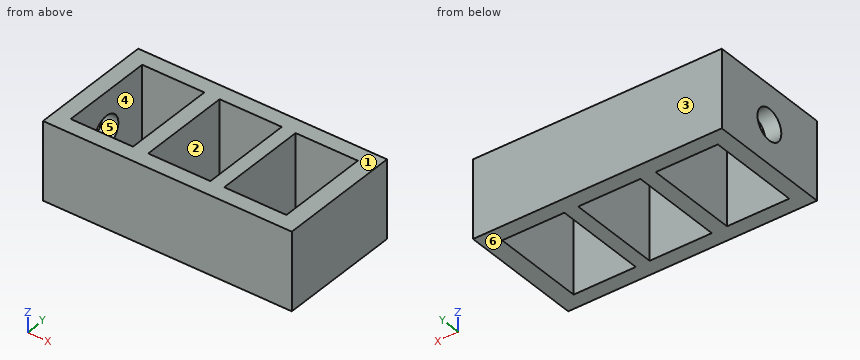
```python
from build123d import *

# Parameters (mm, degrees)
SKETCH_W     = 160
SKETCH_H     = 80
SKETCH_W_2   = 40
SKETCH_H_2   = 60
PAD_DEPTH    = 50
SKETCH001_R  = 10
POCKET_DEPTH = 11


with BuildPart() as part:
    # Sketch → Pad (new body)
    with BuildSketch(Plane.XY):
        Rectangle(SKETCH_W, SKETCH_H)
        with Locations((-49.803748, 0)):
            Rectangle(SKETCH_W_2, SKETCH_H_2, mode=Mode.SUBTRACT)
        Rectangle(SKETCH_W_2, SKETCH_H_2, mode=Mode.SUBTRACT)
        with Locations((48.892394, 0)):
            Rectangle(SKETCH_W_2, SKETCH_H_2, mode=Mode.SUBTRACT)
    extrude(amount=PAD_DEPTH)

    # Sketch001 (on Face1 of Pad) → Pocket (cut)
    with BuildSketch(Plane(origin=(-80, 0, 0), x_dir=(0, -1, 0), z_dir=(-1, 0, 0))):
        with Locations((0, 25)):
            Circle(SKETCH001_R)
    extrude(amount=-POCKET_DEPTH, mode=Mode.SUBTRACT)


solid = part.part
```
For this review, take the finished solid that the model builds, in its own axes (mm). Face numbers are marked on the shaded views. A direction names the side the tool comes from. Round coordinates to 2 decimals unless told otherwise and drop trailing zeros. Order: outer loops, then holes, each group sorted by start corner. A loop starts at its lowest first (then second) coordinate and runs counter-clockwise, first axis right, second up. Notation, with made-up numbers: (68, 76) -> (97, 76) arc R20 ccw to (97, 99) -> close; hole circle Ø9 at (16, -35.75). An arc over 180 degrees is marked (long way). Use a Markdown table: item, result.
Item 1: Draft analysis for pull direction Y (two halves, no side actions). For the marked faces 1, 2 and 3, state which applies: +Y half, -Y half, draft (parallel to the pull), parting line (faces both ways), or undercut.
Resolved:
| item | result |
|---|---|
| face 1 | draft |
| face 2 | undercut |
| face 3 | +Y half |
Item 2: For line 1 along X through (y, z) = (8.5, 43.5); line 2 along X through (y, z) = (0, 25.5); line 3 along Y through (x, z) = (31, 17), list the stretches that pass through material, from the lowest coordinate up. Write a range as [from, to].
Resolved:
| item | result |
|---|---|
| line 1 | x = [-80, -69.8], [-29.8, -20], [20, 28.89], [68.89, 80] |
| line 2 | x = [-29.8, -20], [20, 28.89], [68.89, 80] |
| line 3 | y = [-40, -30], [30, 40] |
Item 3: Take a section at D-D (x = -63.5). State the section outline as (y, z) points.
Resolved:
| item | result |
|---|---|
| outline | (-40, 0) -> (-30, 0) -> (-30, 50) -> (-40, 50) -> close; (30, 0) -> (40, 0) -> (40, 50) -> (30, 50) -> close |
Item 4: Take a section at A-A (z = 12). State the section outline as (x, y) points, plus the area to 3 significant figures.
Resolved:
| item | result |
|---|---|
| outline | (-80, -40) -> (80, -40) -> (80, 40) -> (-80, 40) -> close; hole (-69.8, -30) -> (-29.8, -30) -> (-29.8, 30) -> (-69.8, 30) -> close; hole (-20, -30) -> (20, -30) -> (20, 30) -> (-20, 30) -> close; hole (28.89, -30) -> (68.89, -30) -> (68.89, 30) -> (28.89, 30) -> close |
| area | 5,600 mm² |
Item 5: For pin 1 (8 mm diameter, centred on x = 36, y = 19, fed in from +Z), flat-tipped, find the tip position at first contact; note if it passes through.
Resolved:
| item | result |
|---|---|
| pin 1 | passes through |
Item 6: Take a section at B-B (y = -18). State the section outline as (x, z) points, plus the area to 3 significant figures.
Resolved:
| item | result |
|---|---|
| outline | (-80, 0) -> (-69.8, 0) -> (-69.8, 50) -> (-80, 50) -> close; (-29.8, 0) -> (-20, 0) -> (-20, 50) -> (-29.8, 50) -> close; (20, 0) -> (28.89, 0) -> (28.89, 50) -> (20, 50) -> close; (68.89, 0) -> (80, 0) -> (80, 50) -> (68.89, 50) -> close |
| area | 2,000 mm² |
Item 7: Machinability: for the marked faces 4, 5 and 6, which of the approach directions +Z, -Z, +X, -X, +Y, -Y give a long, thin tool a straight path to every point of the face, cutting with its end or side? Answer none if there is none.
Resolved:
| item | result |
|---|---|
| face 4 | +Z, -Z |
| face 5 | -X |
| face 6 | -Z, +X, -X, +Y, -Y |
Item 8: Take a section at C-C (z = 25). State the section outline as (x, y) points, plus the area to 3 significant figures.
Resolved:
| item | result |
|---|---|
| outline | (-80, -40) -> (80, -40) -> (80, 40) -> (-80, 40) -> (-80, 10) -> (-69.8, 10) -> (-69.8, 30) -> (-29.8, 30) -> (-29.8, -30) -> (-69.8, -30) -> (-69.8, -10) -> (-80, -10) -> close; hole (-20, -30) -> (20, -30) -> (20, 30) -> (-20, 30) -> close; hole (28.89, -30) -> (68.89, -30) -> (68.89, 30) -> (28.89, 30) -> close |
| area | 5,400 mm² |
